Could you check a few things on this drawing? It's one solid part, dimensions in mm from its lowest x, y, z. Coordinates: 2 decimals unless noted, no trailing zeros. Order: outer loops, then holes, each group sorted by start corner. A loop starts at its lowest first (then second) coordinate and runs counter-clockwise, first axis right, second up. Notation, with made-up numbers: (-15.5, 37.25) - (-4.5, 37.25) arc R18 ccw to (-4.5, 63.25) - close; hole circle Ø10 at (60.25, 58). An arc over 180 degrees is marked (long way). Return JSON: item names as keys, results as strings. Group by question number.
1) Imagine slicing it at B-B (y = 1.9). Give the number of separate pieces and of enclosed holes in the cut face, and give its area (3 significant figures).
2) Imagine slicing it at D-D (z = 34). Write out the boundary of the cut face in (x, y).
3) Imagine slicing it at A-A (x = 27.5). Write out the boundary of the cut face in (y, z), and give its area (3 significant figures).
4) If I drill on line 1 along X through (y, z) = (1.85, 26.5); line 2 along X through (y, z) = (0.6, 32) (1 decimal); line 3 along Z through (x, y) = (10, 2) (1 decimal), over which ranges is the centre line in solid material (lowest first)?
5) Imagine slicing it at C-C (x = 46). Write out the boundary of the cut face in (y, z).
6) For pin 1 Ø2.5 at (x, z) = (3.2, 27.5) entering from -Y; pin 2 Ø3 at (x, z) = (46, 27.5) entering from -Y, each with a flat end and sliding along its axis, tell me the tip position at first contact or that it passes through.
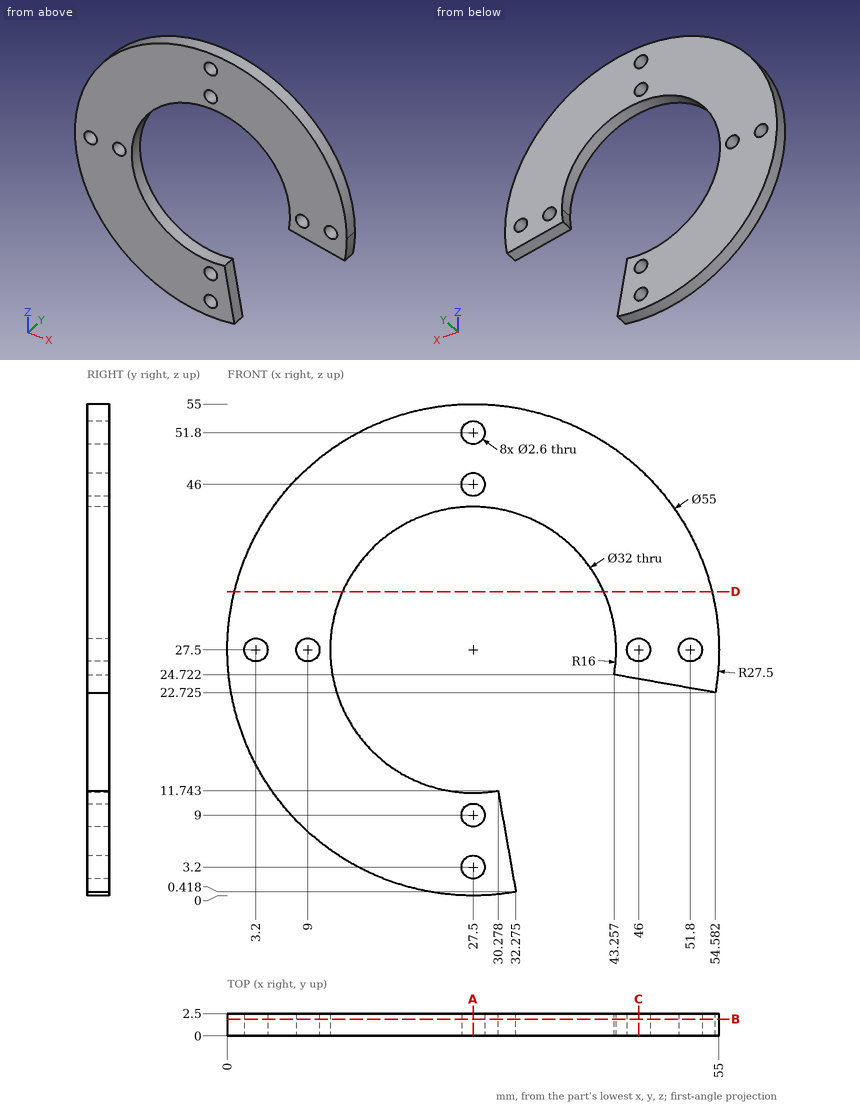
Calculated:
{
 "1": {"separate pieces": "1", "enclosed holes": "8", "area": "1,220 mm2"},
 "2": {"outline": "(0.78, 0) - (12.88, 0) - (12.88, 2.5) - (0.78, 2.5) - close; (42.12, 0) - (54.22, 0) - (54.22, 2.5) - (42.12, 2.5) - close"},
 "3": {"outline": "(0, 0) - (2.5, 0) - (2.5, 1.9) - (0, 1.9) - close; (0, 4.5) - (2.5, 4.5) - (2.5, 7.7) - (0, 7.7) - close; (0, 10.3) - (2.5, 10.3) - (2.5, 11.5) - (0, 11.5) - close; (0, 43.5) - (2.5, 43.5) - (2.5, 44.7) - (0, 44.7) - close; (0, 47.3) - (2.5, 47.3) - (2.5, 50.5) - (0, 50.5) - close; (0, 53.1) - (2.5, 53.1) - (2.5, 55) - (0, 55) - close", "area": "31.5 mm2"},
 "4": {"line 1": "0.02 to 2.37, 4.03 to 8.17, 9.83 to 11.53, 43.47 to 45.17, 46.83 to 50.97, 52.63 to 54.98", "line 2": "0.4 to 12.1, 42.9 to 54.6", "line 3": "6.3 to 26.7, 28.3 to 48.7"},
 "5": {"outline": "(0, 24.24) - (2.5, 24.24) - (2.5, 26.2) - (0, 26.2) - close; (0, 28.8) - (2.5, 28.8) - (2.5, 47.85) - (0, 47.85) - close"},
 "6": {"pin 1": "through", "pin 2": "y = 0"}
}
